Design review of the part built by this model. Coordinates are the model's own, in mm. Face numbers are marked on the shaded views. Give positions to 0.01 mm unless a question says otherwise; leave off trailing zeros. Write each loop counter-clockwise with the first axis right and the second up, starting at its lowest first coordinate (ties: lowest second). Pieces come first, ordered by that corner, then holes.
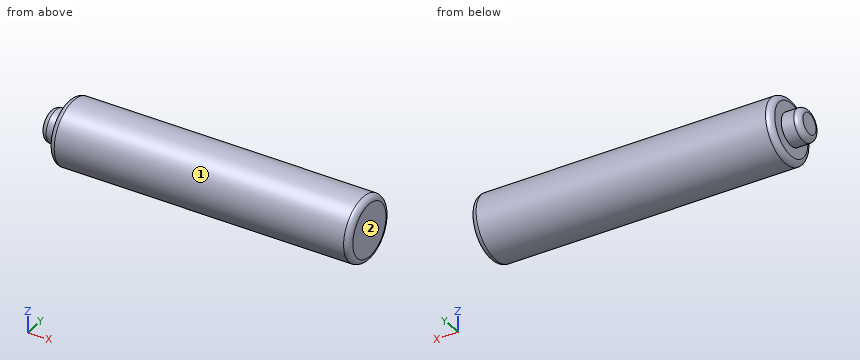
```python
from build123d import *

# Parameters (mm, degrees)
FILLET2_R = 0.762


with BuildPart() as part:
    # Sketch1 → Revolve1 (revolve)
    with BuildSketch(Plane(origin=(0, 0, 0), x_dir=(1, 0, 0), z_dir=(0, 1, 0))):
        Polygon((-45.844442062, 21.494886281), (-5.451340986, 21.494886281), (-5.451340986, 17.215205983), (-45.844442062, 17.215205983), (-48.285381023, 17.215205983), (-48.285381023, 19.355046132), (-45.844442062, 19.355046132), align=None)
    revolve(axis=Axis((-45.844442062, 0, -17.215205983), (1, 0, 0)))

    # Fillet2
    fillet2_edges = [part.edges().sort_by_distance(p)[0] for p in [
        (-48.285381023, 0, -15.075365834),
        (-5.451340986, 0, -12.935525685),
        (-45.844442062, 0, -12.935525685),
    ]]
    fillet(fillet2_edges, radius=FILLET2_R)


solid = part.part
```
(1) To check wall thickness, follow L1, parallel to Y at x = -10.5, z = -17.5; L2, parallel to X at y = 2.5, z = -15.25; L3, parallel to Z at x = -18, y = -0.25. State the ranges of each line that lie inside material, in increasing order.
Resolved:
L1: y = -4.27 to 4.27
L2: x = -45.84 to -5.45
L3: z = -21.49 to -12.94
(2) Clearance check with flat-ended pins moving along their axes: P1, Ø4, axis at y = 3, z = -19.5, coming from the -X side; P2, Ø2, axis at x = -17, z = -15, coming from the +Y side; P3, Ø5, axis at x = -32, y = 3, coming from the -Z side. State where each tip first meets the part, or that it passes through.
Resolved:
P1: stops at x = -48.18
P2: stops at y = 4.1
P3: stops at z = -21.47
(3) Mouldability with a two-part tool opening along Y and no side actions: class the marked faces 1 and 2 as pulls with the +Y half, pulls with the -Y half, needs draft (parallel to the pull), parting line crosses it, or undercut.
Resolved:
face 1: parting line crosses it
face 2: needs draft
(4) Consider section B-B, the plane x = -42.5. Give the boundary of the cut face in (y, z), then the cut area to 3 significant figures.
Resolved:
outline: circle Ø8.56 at (0, -17.22)
area: 57.5 mm2
(5) Consider section A-A, the plane y = 0. Give the boundary of the cut face in (x, z), then the cut area to 3 significant figures.
Resolved:
outline: (-48.29, -18.59) arc R0.76 ccw to (-47.52, -19.36) - (-45.84, -19.36) - (-45.84, -20.73) arc R0.76 ccw to (-45.08, -21.49) - (-6.21, -21.49) arc R0.76 ccw to (-5.45, -20.73) - (-5.45, -13.7) arc R0.76 ccw to (-6.21, -12.94) - (-45.08, -12.94) arc R0.76 ccw to (-45.84, -13.7) - (-45.84, -15.08) - (-47.52, -15.08) arc R0.76 ccw to (-48.29, -15.84) - close
area: 355 mm2
